from build123d import *

# Parameters (mm, degrees)
F1_DEPTH = 23
F2_DEPTH = 23
F3_R     = 11
F4_DEPTH = 25
F5_R     = 1


with BuildPart() as f1:
    # F0 (on Front) → F1 (new body)
    with BuildSketch(Plane.XZ):
        Polygon((2.5250660033, -1.4578475367), (5, 0), (2.5, 4.3301270189), (0, 2.9156950735), (-2.5, 4.3301270189), (-5, 0), (-2.5250660033, -1.4578475367), (-2.5, -4.3301270189), (2.5, -4.3301270189), align=None)
    extrude(amount=F1_DEPTH)

    # F0 (on Front) → F2 (join, through all)
    with BuildSketch(Plane.XZ):
        with BuildLine():
            Line((2.5, 4.3301270189), (5, 0))
            ThreePointArc((5, 0), (4.3301270189, 2.5), (2.5, 4.3301270189))
        make_face()
        with BuildLine():
            Line((-5, 0), (-2.5, 4.3301270189))
            ThreePointArc((-2.5, 4.3301270189), (-4.3301270189, 2.5), (-5, 0))
        make_face()
        with BuildLine():
            ThreePointArc((-2.5, -4.3301270189), (0, -5), (2.5, -4.3301270189))
            Line((2.5, -4.3301270189), (-2.5, -4.3301270189))
        make_face()
    extrude(amount=F2_DEPTH)

    # F3 (on face) → F4 (join)
    with BuildSketch(Plane.XZ.offset(23)):
        Circle(F3_R)
        with BuildLine():
            Line((5, 0), (2.5250660033, -1.4578475367))
            Line((2.5250660033, -1.4578475367), (2.5, -4.3301270189))
            ThreePointArc((2.5, -4.3301270189), (0, -5), (-2.5, -4.3301270189))
            Line((-2.5, -4.3301270189), (-2.5250660033, -1.4578475367))
            Line((-2.5250660033, -1.4578475367), (-5, 0))
            ThreePointArc((-5, 0), (-4.3301270189, 2.5), (-2.5, 4.3301270189))
            Line((-2.5, 4.3301270189), (0, 2.9156950735))
            Line((0, 2.9156950735), (2.5, 4.3301270189))
            ThreePointArc((2.5, 4.3301270189), (4.3301270189, 2.5), (5, 0))
        make_face(mode=Mode.SUBTRACT)
        with BuildLine():
            Line((2.5, -4.3301270189), (2.5250660033, -1.4578475367))
            Line((2.5250660033, -1.4578475367), (5, 0))
            ThreePointArc((5, 0), (4.3301270189, 2.5), (2.5, 4.3301270189))
            Line((2.5, 4.3301270189), (0, 2.9156950735))
            Line((0, 2.9156950735), (-2.5, 4.3301270189))
            ThreePointArc((-2.5, 4.3301270189), (-4.3301270189, 2.5), (-5, 0))
            Line((-5, 0), (-2.5250660033, -1.4578475367))
            Line((-2.5250660033, -1.4578475367), (-2.5, -4.3301270189))
            ThreePointArc((-2.5, -4.3301270189), (0, -5), (2.5, -4.3301270189))
        make_face()
    extrude(amount=F4_DEPTH)

    # F5
    f5_edges = [f1.edges().sort_by_distance(p)[0] for p in [
        (-11, -23, 0),
        (3.762533, -23, -0.728924),
        (4.330127, -23, 2.5),
        (1.25, -23, 3.622911),
        (-1.25, -23, 3.622911),
        (-4.330127, -23, 2.5),
        (-3.762533, -23, -0.728924),
        (-2.512533, -23, -2.893987),
        (0, -23, -5),
        (2.512533, -23, -2.893987),
    ]]
    fillet(f5_edges, radius=F5_R)


solid = f1.part
Work out the finished part from the listing and answer in its coordinate system (mm). A direction names the side the tool comes from. Round coordinates to 2 decimals unless told otherwise and drop trailing zeros. Write each loop counter-clockwise with the first axis right and the second up, starting at its lowest first coordinate (ties: lowest second). Pieces come first, ordered by that corner, then holes. Notation, with made-up numbers: (1.5, -0.75) - (14.5, -0.75) arc R30 ccw to (14.5, 36.25) - close; hole circle Ø9 at (62.25, 88.25). An arc over 180 degrees is marked (long way). Answer in a Markdown table with one row per item. Add a question column.
1. Find the intervals of material crossed by line 1 along Y through (x, z) = (-6.5, -1.75); line 2 along X through (y, z) = (-11.5, 4); line 3 along X through (y, z) = (-3, -1.75), in increasing order. Write a range as from..to.
2. The mould has two halves that part along X. Classify faces 4 (the cylindrical face through (1.315, -22.715, 4.005)), 5 (the cylindrical face through (-2.38, -35.83, -10.74)), 6 (the flat face through (0, 0, 0)), 7 (the flat face through (1.267, -10.846, 3.633)): +X half, -X half, draft (parallel to the pull), parting line (faces both ways), or undercut.
3. Given pin 1 (5 mm diameter, centred on y = -21.5, z = -8, fed in from +X); pin 2 (8 mm diameter, centred on y = -17.5, z = -6, fed in from -X); pin 3 (1.5 mm diameter, centred on x = -4, y = -17, fed in from -Z), each flat-ended and moving along its own axis, determine where each tip first touches the part or whether it passes through.
4. For faces 1 (the cylindrical face through (4.348, -10.846, 2.468)), 2 (the cylindrical face through (-4, -11, 3)), 3 (the cylindrical face through (0, -11, -5)), determine the directions among +Z, -Z, +X, -X, +Y, -Y from which every point of the face is accessible in a straight line to the end or side of a thin tool.
5. A cutting plane is placed at A-A, the plane y = -21. Determine the outline of the cut face in (x, z), and give its area (3 significant figures).
Worked out:
| question | item | result |
|---|---|---|
| 1 | line 1 | -48..-23 |
| 1 | line 2 | -3..-1.92, 1.92..3 |
| 1 | line 3 | -2.52..2.52 |
| 2 | face 4 | undercut |
| 2 | face 5 | parting line |
| 2 | face 6 | draft |
| 2 | face 7 | undercut |
| 3 | pin 1 | x = 8.72 |
| 3 | pin 2 | x = -2.52 |
| 3 | pin 3 | z = -1.03 |
| 4 | face 1 | +Z, +X, +Y |
| 4 | face 2 | +Z, -X, +Y |
| 4 | face 3 | -Z, +Y |
| 5 | outline | (-5, 0) - (-2.53, -1.46) - (-2.5, -4.33) arc R5 ccw to (2.5, -4.33) - (2.53, -1.46) - (5, 0) arc R5 ccw to (2.5, 4.33) - (0, 2.92) - (-2.5, 4.33) arc R5 ccw to start |
| 5 | area | 61.1 mm^2 |
